Geometry: see drawing. Coordinates: mm, zero at the bounding-box minimum. A direction names the side the tool comes from. Round coordinates to 2 decimals unless told otherwise and drop trailing zeros. Loops run counter-clockwise (first coordinate to the right, second up) from the corner with the lowest first, then second, coordinate; pieces in that order, holes last.
(1) Cut plane A-A, the plane x = 17.5. Output: boundary loops of the cut face in (y, z).
(2) Access query for the marked faces 4 and 5. Directions: +Z, -Z, +X, -X, +Y, -Y. A direction counts if a zero-diameter tool reaches every point of the face in a straight line with its end or side. Return the directions, or none.
(3) Draft query along Y for the marked faces 1, 2 and 3. Return one class per face: released by +Y, released by -Y, zero draft, split by the parting line, or undercut.
(4) Cut plane B-B, the plane z = 10.75. Output: boundary loops of the cut face in (x, y).
(5) Cut plane C-C, the plane z = 8.25. Output: boundary loops of the cut face in (x, y).
(6) Line query: line 1 (Y direction, x = 17.5, z = 3.5); line 2 (Y direction, x = 23, z = 11.5) (1 decimal); line 3 (X direction, y = 17, z = 14) (1 decimal). Output: solid intervals per line, ascending.
(7) First-contact query: pin 1 Ø6 at (x, y) = (17.5, 17.5) entering from +Z; pin 2 Ø2 at (x, z) = (9.5, 11.5) entering from +Y; pin 3 Ø4 at (y, z) = (12, 10.5) entering from +X; pin 4 Ø3 at (x, z) = (4, 2) entering from -Y. Flat tips, straight axial feed; report the tip coordinate or a pass-through.
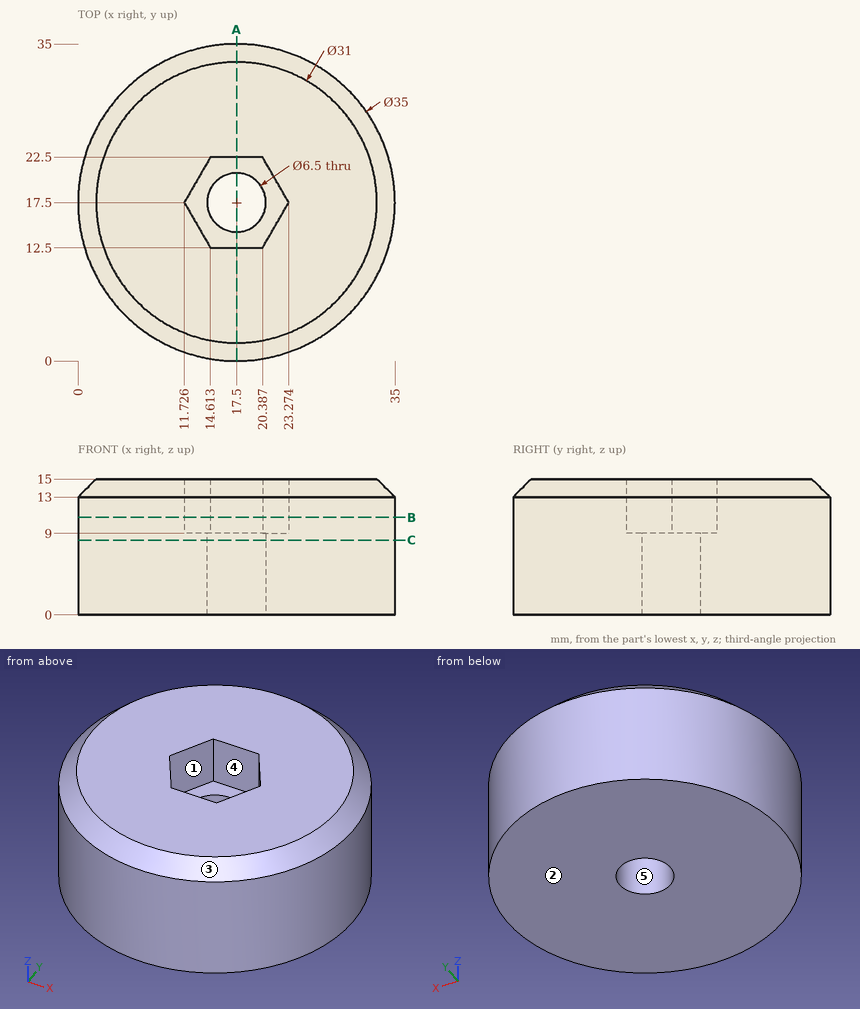
Reported:
1. outline: (0, 0) - (14.25, 0) - (14.25, 9) - (12.5, 9) - (12.5, 15) - (2, 15) - (0, 13) - close; (20.75, 0) - (35, 0) - (35, 13) - (33, 15) - (22.5, 15) - (22.5, 9) - (20.75, 9) - close
2. face 4: +Z
2. face 5: +Z, -Z
3. face 1: undercut
3. face 2: zero draft
3. face 3: split by the parting line
4. outline: circle Ø35 at (17.5, 17.5); hole (11.73, 17.5) - (14.61, 12.5) - (20.39, 12.5) - (23.27, 17.5) - (20.39, 22.5) - (14.61, 22.5) - close
5. outline: circle Ø35 at (17.5, 17.5); hole circle Ø6.5 at (17.5, 17.5)
6. line 1: y = 0 to 14.25, 20.75 to 35
6. line 2: y = 0.9 to 17, 18 to 34.1
6. line 3: x = 1 to 12, 23 to 34
7. pin 1: passes through
7. pin 2: stops at y = 33.54
7. pin 3: stops at x = 34.65
7. pin 4: stops at y = 4.76
